Check sheet for the modelled part. Datum: model origin and axes. Units: mm. A direction names the side the tool comes from. Coordinates: 2 decimals unless noted, no trailing zeros. Loops run counter-clockwise (first coordinate to the right, second up) from the corner with the lowest first, then second, coordinate; pieces in that order, holes last. Notation, with made-up numbers: M 82,-15 L 122,-15 A24 ccw 122,1 Z; hole C -33,-22.5 d6. An arc over 180 degrees is marked long. Return JSON: item names as keys, results as strings.
from build123d import *

# Parameters (mm, degrees)
F0_W           = 254
F0_H           = 50.8
F1_DEPTH       = 50.8
F3_D           = 13.4874
F3_DEPTH       = 25.4
F3_CBORE_D     = 20.6375
F3_CBORE_DEPTH = 17.78
F5_D           = 13.4874
F5_DEPTH       = 25.4
F5_CBORE_D     = 20.6375
F5_CBORE_DEPTH = 17.78


with BuildPart() as f1:
    # F0 (on Front) → F1 (new body)
    with BuildSketch(Plane.XZ):
        Rectangle(F0_W, F0_H)
    extrude(amount=F1_DEPTH)

    # F3
    with Locations(Plane(origin=(0, 0, 0), x_dir=(-1, 0, 0), z_dir=(0, 1, 0))):
        with Locations((-63.5, 0), (63.5, 0)):
            CounterBoreHole(F3_D / 2, F3_CBORE_D / 2, F3_CBORE_DEPTH, depth=F3_DEPTH)

    # F5
    with Locations(Plane.XZ.offset(50.8)):
        with Locations((-63.5, 0), (63.5, 0)):
            CounterBoreHole(F5_D / 2, F5_CBORE_D / 2, F5_CBORE_DEPTH, depth=F5_DEPTH)


solid = f1.part
1) Go/stop test with flat-tipped pins: pin 1 Ø8 at (x, z) = (-63.5, 0) entering from +Y; pin 2 Ø10.5 at (x, z) = (-61, 3) entering from -Y; pin 3 Ø17.5 at (x, z) = (63.5, 0) entering from +Y. Record where each tip stops, or that it passes through.
Answers:
{"pin 1": "through", "pin 2": "y = -33.02", "pin 3": "y = -17.78"}
2) Section check B-B on x = 63.5. Record the cut outline in (y, z).
Answers:
{"outline": "M -50.8,-25.4 L 0,-25.4 L 0,-10.32 L -17.78,-10.32 L -17.78,-6.74 L -33.02,-6.74 L -33.02,-10.32 L -50.8,-10.32 Z; M -50.8,10.32 L -33.02,10.32 L -33.02,6.74 L -17.78,6.74 L -17.78,10.32 L 0,10.32 L 0,25.4 L -50.8,25.4 Z"}
3) Section check C-C on y = -11.5. Record the cut outline in (x, z), then the cut area to 3 significant figures.
Answers:
{"outline": "M -127,-25.4 L 127,-25.4 L 127,25.4 L -127,25.4 Z; hole C -63.5,0 d20.64; hole C 63.5,0 d20.64", "area": "12,200 mm²"}
4) Draft check along X on faces 4 (the face through (61, -17.78, -7)), 5 (the face through (-73.032, -8.766, -3.952)), 6 (the face through (127, -25, 0)), 7 (the face through (-2, 0, 0)). Enter one of: +X half, -X half, draft (parallel to the pull), parting line (faces both ways), or undercut.
Answers:
{"face 4": "undercut", "face 5": "undercut", "face 6": "+X half", "face 7": "draft"}
5) Section check A-A on z = 0. Record the cut outline in (x, y).
Answers:
{"outline": "M -127,-50.8 L -73.82,-50.8 L -73.82,-33.02 L -70.24,-33.02 L -70.24,-17.78 L -73.82,-17.78 L -73.82,0 L -127,0 Z; M -56.76,-33.02 L -53.18,-33.02 L -53.18,-50.8 L 53.18,-50.8 L 53.18,-33.02 L 56.76,-33.02 L 56.76,-17.78 L 53.18,-17.78 L 53.18,0 L -53.18,0 L -53.18,-17.78 L -56.76,-17.78 Z; M 70.24,-33.02 L 73.82,-33.02 L 73.82,-50.8 L 127,-50.8 L 127,0 L 73.82,0 L 73.82,-17.78 L 70.24,-17.78 Z"}
6) Set-up check for faces 1 (the face through (-66, -17.78, -7)), 2 (the face through (-61, -33.02, -7)), 3 (the face through (-2, -50.8, 0)): record each of +Z, -Z, +X, -X, +Y, -Y from which the full face is reachable in a straight line by a thin tool's end or side.
Answers:
{"face 1": "+Y", "face 2": "-Y", "face 3": "+Z, -Z, +X, -X, -Y"}
7) Scan lines: line 1 along X through (y, z) = (-28.25, 0); line 2 along Z through (x, y) = (63.5, -38); line 3 along X through (y, z) = (-42.5, 3). Record each from-to range of solid material in increasing order. Write a range as [from, to].
Answers:
{"line 1": "[-127, -70.24], [-56.76, 56.76], [70.24, 127]", "line 2": "[-25.4, -10.32], [10.32, 25.4]", "line 3": "[-127, -73.37], [-53.63, 53.63], [73.37, 127]"}
